```python
from build123d import *

# Parameters (mm, degrees)
SKETCH1_R           = 38.1
SKETCH1_R_2         = 4
BOSS_EXTRUDE2_DEPTH = 3.175
SKETCH4_R           = 2.25
CUT_EXTRUDE3_DEPTH  = 30.394


with BuildPart() as part:
    # Sketch1 → Boss-Extrude2 (new body)
    with BuildSketch(Plane.YZ):
        with Locations(Location((0, 0, 0), (0, 0, 270))):
            Circle(SKETCH1_R)
        with Locations(Location((0, 0, 0), (0, 0, 270))):
            Circle(SKETCH1_R_2, mode=Mode.SUBTRACT)
    extrude(amount=BOSS_EXTRUDE2_DEPTH)

    # Sketch4 → Cut-Extrude3 (cut)
    with BuildSketch(Plane.YZ.offset(3.175)):
        with Locations(Location((0, 11.313708499, 0), (0, 0, 270))):
            Circle(SKETCH4_R)
        with Locations(Location((11.313708499, 0, 0), (0, 0, 270))):
            Circle(SKETCH4_R)
        with Locations(Location((-11.313708499, 0, 0), (0, 0, 270))):
            Circle(SKETCH4_R)
        with Locations(Location((0, -11.313708499, 0), (0, 0, 270))):
            Circle(SKETCH4_R)
    extrude(amount=-CUT_EXTRUDE3_DEPTH, mode=Mode.SUBTRACT)


solid = part.part
```
Model file for the job. Use its own axes, mm. Coordinates: 2 decimals unless noted, no trailing zeros. Loops run counter-clockwise (first coordinate to the right, second up) from the corner with the lowest first, then second, coordinate; pieces in that order, holes last. Notation, with made-up numbers: (19.25, 56.5) - (28.25, 56.5) arc R8 ccw to (28.25, 64.5) - close; hole circle Ø8 at (85, 11). An arc over 180 degrees is marked (long way). Write item = value, one per line. Start each with the question number.
Item 1: Saw through at A-A, the plane y = 0. List the corners of the cut face in (x, z) (3 decimals).
Item 2: Wall check: probe 1 along Z at (x, y) = (2.8, 12); probe 2 along Y at (x, z) = (2.1, 3); probe 3 along Z at (x, y) = (2.6, -11). Give the ranges that are in metal, low to high. Write a range as [from, to].
Item 3: Pull direction Z, two halves, no side cores. Call faces 1 (the face through (3.175, 1, -8)), 2 (the face through (1.565, -23.183, 30.235)), 3 (the face through (1.61, 13.21, -1.21)): +Z half, -Z half, draft (parallel to the pull), parting line (faces both ways), or undercut.
Item 4: Drop a flat-ended pin along its axis: pin 1 Ø1.5 at (x, z) = (2, -1.5) entering from -Y. Give the stop position or say it passes through.
Item 5: Saw through at D-D, the plane z = 29.5. List the corners of the cut face in (x, y) (3 decimals), then the cut area to 3 significant figures.
Item 6: Saw through at C-C, the plane x = 2.4. List the corners of the cut face in (y, z), then the cut area to 3 significant figures.
Answers:
q1.outline = (0, -38.1) - (3.175, -38.1) - (3.175, -13.564) - (0, -13.564) - close; (0, -9.064) - (3.175, -9.064) - (3.175, -4) - (0, -4) - close; (0, 4) - (3.175, 4) - (3.175, 9.064) - (0, 9.064) - close; (0, 13.564) - (3.175, 13.564) - (3.175, 38.1) - (0, 38.1) - close
q2.probe_1 = [-36.16, -2.14], [2.14, 36.16]
q2.probe_2 = [-37.98, -2.65], [2.65, 37.98]
q2.probe_3 = [-36.48, -2.23], [2.23, 36.48]
q3.face_1 = draft
q3.face_2 = parting line
q3.face_3 = undercut
q4.pin_1 = -38.09
q5.outline = (0, -24.111) - (3.175, -24.111) - (3.175, 24.111) - (0, 24.111) - close
q5.area = 153 mm2
q6.outline = circle Ø76.2 at (0, 0); hole circle Ø4.5 at (-11.31, 0); hole circle Ø8 at (0, 0); hole circle Ø4.5 at (0, -11.31); hole circle Ø4.5 at (0, 11.31); hole circle Ø4.5 at (11.31, 0)
q6.area = 4,450 mm2
